Part model, mm, in its own coordinate system. A direction names the side the tool comes from. Round coordinates to 2 decimals unless told otherwise and drop trailing zeros. Loops run counter-clockwise (first coordinate to the right, second up) from the corner with the lowest first, then second, coordinate; pieces in that order, holes last.
1) Band-saw the part on A-A, the plane y = 18.5. Write the cut outline in (x, z) (3 decimals).
2) Probe line 1 (Z direction, x = 25.4, y = 2.2); line 2 (X direction, y = 2.35, z = 279.4); line 3 (X direction, y = 12, z = 29.5) (3 decimals). List the from-to ranges inside material, lowest first.
3) Drop a flat-ended pin along its axis: P1, Ø13.5, axis at x = 19, z = 172, coming from the +Y side (3 decimals). Give the stop position or say it passes through.
4) Band-saw the part on B-B, the plane z = 279.4. Write the cut outline in (x, y) (1 decimal).
5) Band-saw the part on C-C, the plane x = 25.4. Write the cut outline in (y, z) (1 decimal).
6) Mould opens along Z. For faces 3 (the flat face through (3.175, 14, 150)), 4 (the flat face through (27, 2, 304.8)), 5 (the cylindrical face through (24.04, 1.61, 269.01)) say: +Z half, -Z half, draft (parallel to the pull), parting line (faces both ways), or undercut.
7) Band-saw the part on D-D, the plane z = 19. Write the cut outline in (x, y) (3 decimals), then the cut area to 3 significant figures.
8) 3-axis set-ups, long thin cutter, end or side, ignore diameter. For faces 1 (the flat face through (50.8, 13, 150)), 2 (the flat face through (47.625, 14, 150)): which of +Z, -Z, +X, -X, +Y, -Y reach the whole face in a straight line?
from build123d import *

# Parameters (mm, degrees)
SKETCH1_W           = 50.8
SKETCH1_H           = 25.4
BOSS_EXTRUDE1_DEPTH = 304.8
SKETCH2_W           = 44.45
SKETCH2_H           = 22.225
CUT_EXTRUDE1_DEPTH  = 305.8
SKETCH3_R           = 10.4775
CUT_EXTRUDE2_DEPTH  = 4.175


with BuildPart() as part:
    # Sketch1 → Boss-Extrude1 (new body)
    with BuildSketch(Plane.XY):
        with Locations((25.4, 12.7)):
            Rectangle(SKETCH1_W, SKETCH1_H)
    extrude(amount=BOSS_EXTRUDE1_DEPTH)

    # Sketch2 → Cut-Extrude1 (cut, through all)
    with BuildSketch(Plane(origin=(0, 0, 0), x_dir=(-1, 0, 0), z_dir=(0, 0, -1))):
        with Locations((-25.4, 14.2875)):
            Rectangle(SKETCH2_W, SKETCH2_H)
    extrude(amount=-CUT_EXTRUDE1_DEPTH, mode=Mode.SUBTRACT)

    # Sketch3 → Cut-Extrude2 (cut, through all)
    with BuildSketch(Plane(origin=(0, 3.175, 0), x_dir=(1, 0, 0), z_dir=(0, 1, 0))):
        with Locations((25.4, -279.4)):
            Circle(SKETCH3_R)
    extrude(amount=-CUT_EXTRUDE2_DEPTH, mode=Mode.SUBTRACT)


solid = part.part
Reported:
1. outline: (0, 0) - (3.175, 0) - (3.175, 304.8) - (0, 304.8) - close; (47.625, 0) - (50.8, 0) - (50.8, 304.8) - (47.625, 304.8) - close
2. line 1: z = 0 to 268.92, 289.88 to 304.8
2. line 2: x = 0 to 14.92, 35.88 to 50.8
2. line 3: x = 0 to 3.175, 47.625 to 50.8
3. P1: stops at y = 3.175
4. outline: (0, 0) - (14.9, 0) - (14.9, 3.2) - (3.2, 3.2) - (3.2, 25.4) - (0, 25.4) - close; (35.9, 0) - (50.8, 0) - (50.8, 25.4) - (47.6, 25.4) - (47.6, 3.2) - (35.9, 3.2) - close
5. outline: (0, 0) - (3.2, 0) - (3.2, 268.9) - (0, 268.9) - close; (0, 289.9) - (3.2, 289.9) - (3.2, 304.8) - (0, 304.8) - close
6. face 3: draft
6. face 4: +Z half
6. face 5: undercut
7. outline: (0, 0) - (50.8, 0) - (50.8, 25.4) - (47.625, 25.4) - (47.625, 3.175) - (3.175, 3.175) - (3.175, 25.4) - (0, 25.4) - close
7. area: 302 mm2
8. face 1: +Z, -Z, +X, +Y, -Y
8. face 2: +Z, -Z, +Y
